Here's how the part is built. I have some questions about the finished solid (model axes, mm). A direction names the side the tool comes from. Give positions to 0.01 mm unless a question says otherwise; leave off trailing zeros. Write each loop counter-clockwise with the first axis right and the second up, starting at its lowest first coordinate (ties: lowest second). Pieces come first, ordered by that corner, then holes. Notation, with made-up numbers: M 30,0.25 L 45,0.25 A30 cw 45,35.25 Z; hole C 75.5,40 d3. An arc over 180 degrees is marked long. Answer as CSV lines item,"result". Start each with the question number.
Q1. Thinking about a two-plate mould opening in X: for faces 1 (the flat face through (-9, 1, 0)), 2 (the flat face through (9, 1, 0)), 3 (the flat face through (0, 2, 0)), 4 (the flat face through (8, 0, 2)), which applies, +X half, -X half, draft (parallel to the pull), parting line (faces both ways), or undercut?
Q2. Suppose I cut it at C-C (y = -6). Write out the boundary of the cut face in (x, z).
Q3. On a 3-axis mill with a long thin cutter (end or side, diameter ignored), from which of +Z, -Z, +X, -X, +Y, -Y can I reach the whole of each face in a straight line? I mean faces 5 (the flat face through (-8.236, 3.497, 8.117)), 6 (the cylindrical face through (-1.487, -10.195, -4.958)), 7 (the cylindrical face through (0.1, -10.1, 2.5)). Say none if no direction works.
Q4. Suppose I cut it at A-A (x = 0). Write out the boundary of the cut face in (y, z), then the cut area to 4 significant figures.
Q5. Suppose I cut it at B-B (z = 0). Write out the boundary of the cut face in (x, y), then the cut area to 3 significant figures.
Q6. Suppose I cut it at D-D (z = -3.25). Write out the boundary of the cut face in (x, y).
Q7. If I drill on line 1 along X through (y, z) = (-12.75, 0); line 2 along Y through (x, z) = (0, -3.75); line 3 along Y through (x, z) = (-2.75, -3.5), over which ranges is the centre line in solid material (lowest first)?
Q8. For pin 1 (4 mm diameter, centred on x = 5.5, z = -3.5, fed in from +Y); pin 2 (5 mm diameter, centred on y = -4, z = 7, fed in from -X); pin 3 (5 mm diameter, centred on x = -2.5, y = -13, fed in from +Z), each with a flat end and sliding along its axis, tell me the tip position at first contact or that it passes through.
```python
from build123d import *

# Parameters (mm, degrees)
SKETCH1_W           = 18
SKETCH1_H           = 18
BOSS_EXTRUDE1_DEPTH = 2
BOSS_EXTRUDE2_DEPTH = 3
CUT_EXTRUDE4_DEPTH  = 3
SKETCH5_R           = 8
BOSS_EXTRUDE3_DEPTH = 20
SKETCH6_R           = 2.5
CUT_EXTRUDE5_DEPTH  = 20
SKETCH7_R           = 1.5
CUT_EXTRUDE6_DEPTH  = 20


# Read off the part's stored shape, not the designer's step: Mirror1, Mirror2
with BuildPart() as part:
    # Sketch1 → Boss-Extrude1 (new body)
    with BuildSketch(Plane(origin=(0, 0, 0), x_dir=(1, 0, 0), z_dir=(0, 1, 0))):
        Rectangle(SKETCH1_W, SKETCH1_H)
    extrude(amount=BOSS_EXTRUDE1_DEPTH)

    # Sketch2 → Boss-Extrude2 (add)
    with BuildSketch(Plane(origin=(0, 2, 0), x_dir=(1, 0, 0), z_dir=(0, 1, 0))):
        Polygon((-9, 9), (-7, 9), (-9, 7), align=None)
        Polygon((9, 7), (9, 9), (7, 9), align=None)
        Polygon((7, -9), (9, -7), (9, -9), align=None)
        Polygon((-9, -7), (-9, -9), (-7, -9), align=None)
    extrude(amount=BOSS_EXTRUDE2_DEPTH)

    # Sketch4 → Cut-Extrude4 (cut)
    with BuildSketch(Plane(origin=(-7.554451855, -1.780601378, -7.554451855), x_dir=(0.7165985720844784, -0.16001422411879979, -0.678882857764243), z_dir=(0.697485832462916, 0.16439898730535757, 0.6974858324629155))):
        Polygon((-2.017235593, 6.634774192), (-2.017235593, 3.552567191), (0.773727267, 4.011398658), (-0.213027115, 6.931384239), align=None)
    extrude(amount=CUT_EXTRUDE4_DEPTH, mode=Mode.SUBTRACT)


with BuildPart() as cut_extrude4_kept_piece:
    # of the separate pieces the step leaves, the one the design keeps (cut_extrude4_pieces_kept)
    add(part.part.solids().sort_by_distance((-9, 0, -9))[0])

    # Mirror1
    split(bisect_by=Plane(origin=(0, 0, 0), x_dir=(0, 0, 1), z_dir=(1, 0, 0)), keep=Keep.BOTTOM)

    # Mirror1 2: Cut-Extrude4 kept piece across plane


with BuildPart() as cut_extrude4_kept_piece_1:
    add(cut_extrude4_kept_piece.part)
    add(cut_extrude4_kept_piece.part.mirror(Plane(origin=(0, 0, 0), x_dir=(0, 0, 1), z_dir=(1, 0, 0))))

    # Mirror2
    split(bisect_by=Plane.XY, keep=Keep.BOTTOM)

    # Mirror2 2: Cut-Extrude4 kept piece across plane


with BuildPart() as cut_extrude4_kept_piece_2:
    add(cut_extrude4_kept_piece_1.part)
    add(cut_extrude4_kept_piece_1.part.mirror(Plane.XY))

    # Sketch5 → Boss-Extrude3 (add)
    with BuildSketch(Plane.XZ):
        with Locations(Location((0, 0, 0), (0, 0, 270))):
            Circle(SKETCH5_R)
    extrude(amount=BOSS_EXTRUDE3_DEPTH)

    # Sketch6 → Cut-Extrude5 (cut)
    with BuildSketch(Plane.XZ.offset(20)):
        with Locations(Location((0, 0, 0), (0, 0, 270))):
            Circle(SKETCH6_R)
    extrude(amount=-CUT_EXTRUDE5_DEPTH, mode=Mode.SUBTRACT)

    # Sketch7 → Cut-Extrude6 (cut)
    with BuildSketch(Plane.XY):
        with Locations(Location((0, -10, 0), (0, 0, 90))):
            Circle(SKETCH7_R)
    extrude(amount=-CUT_EXTRUDE6_DEPTH, mode=Mode.SUBTRACT)


solid = cut_extrude4_kept_piece_2.part
```
Resolved:
1,face 1,"-X half"
1,face 2,"+X half"
1,face 3,"undercut"
1,face 4,"draft"
2,outline,"C 0,0 d16; hole C 0,0 d5"
3,face 5,"+Y"
3,face 6,"-Z"
3,face 7,"-Y"
4,outline,"M -20,-8 L -11.5,-8 L -11.5,-2.5 L -20,-2.5 Z; M -20,2.5 L 0,2.5 L 0,-2.5 L -8.5,-2.5 L -8.5,-8 L 0,-8 L 0,-9 L 2,-9 L 2,9 L 0,9 L 0,8 L -20,8 Z"
4,area,"239.5 mm^2"
5,outline,"M -9,0 L -8,0 L -8,-20 L -2.5,-20 L -2.5,0 L 2.5,0 L 2.5,-20 L 8,-20 L 8,0 L 9,0 L 9,2 L -9,2 Z"
5,area,"256 mm^2"
6,outline,"M -9,0 L -7.31,0 L -7.31,-20 L 7.31,-20 L 7.31,0 L 9,0 L 9,2 L -9,2 Z; hole C 0,-10 d3"
7,line 1,"-8 to -2.5, 2.5 to 8"
7,line 2,"-20 to -11.5, -8.5 to 2"
7,line 3,"-20 to 2"
8,pin 1,"y = 2"
8,pin 2,"x = -6.61"
8,pin 3,"z = 8"
